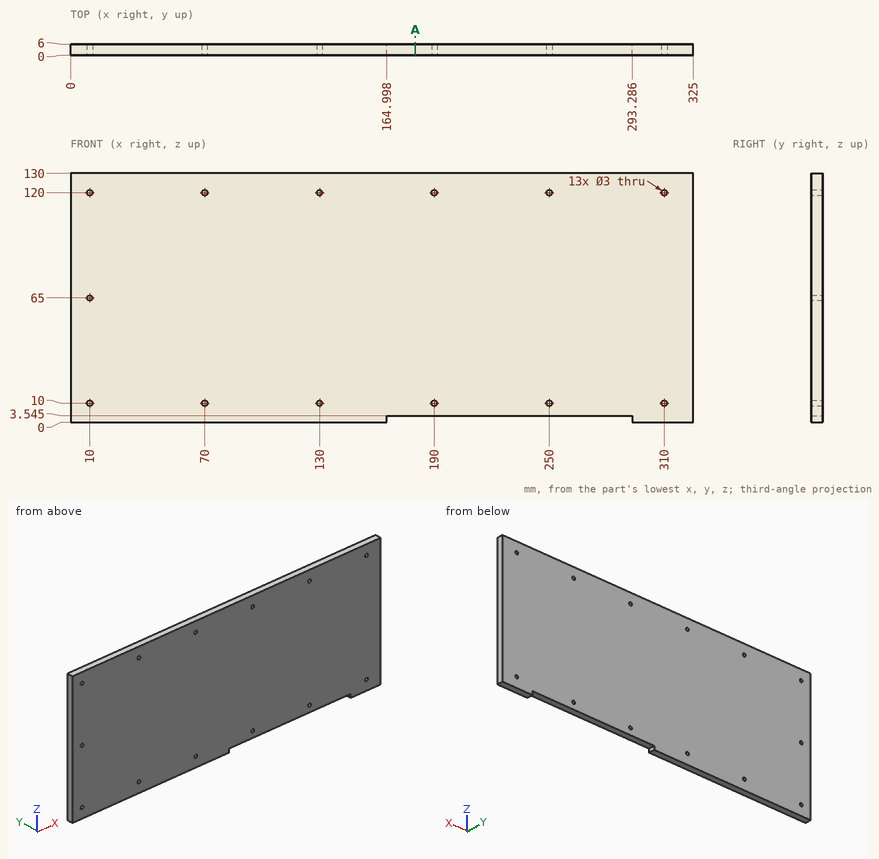
Answer from the drawing. Dimensions are ordinates in mm from the lowest x, y and z of the part. Coordinates: 2 decimals unless noted, no trailing zeros. Loops run counter-clockwise (first coordinate to the right, second up) from the corner with the lowest first, then second, coordinate; pieces in that order, holes last.
1) Consider probe 1 along Z at (x, y) = (310, 2); probe 2 along X at (y, z) = (2.4, 65); probe 3 along Z at (x, y) = (238, 1.5) (1 decimal). Determine where each line is inside the solid, lowest interval first.
Results:
probe 1: z = 0 to 8.5, 11.5 to 118.5, 121.5 to 130
probe 2: x = 0 to 8.5, 11.5 to 325
probe 3: z = 3.5 to 130
2) Section A-A (x = 180) is taken. Give the vertices of the cut face in (y, z) (1 decimal), plus the area to 3 significant figures.
Results:
outline: (0, 3.5) - (6, 3.5) - (6, 130) - (0, 130) - close
area: 759 mm2
3) Flat-ended cylindrical pins translate along their axes: pin 1 (2.5 mm diameter, centred on x = 250, z = 10, fed in from -Y); pin 2 (1.5 mm diameter, centred on x = 272.5, z = 102.5, fed in from -Y); pin 3 (1.8 mm diameter, centred on x = 217.5, y = 4, fed in from -Z) (1 decimal). Find the tip coordinate at first contact, or state that the pin passes through.
Results:
pin 1: passes through
pin 2: stops at y = 0
pin 3: stops at z = 3.5
